The listing builds one solid part. Answer for the finished solid, in the listing's coordinates (mm). A direction names the side the tool comes from. Round coordinates to 2 decimals unless told otherwise and drop trailing zeros. Order: outer loops, then holes, each group sorted by start corner. A loop starts at its lowest first (then second) coordinate and runs counter-clockwise, first axis right, second up. Notation, with made-up numbers: (4.5, -6) - (58.5, -6) arc R13 ccw to (58.5, -2) - close; hole circle Ø1 at (-27, 4.5). An arc over 180 degrees is marked (long way). Use CSV: the item, a comma, the result in double quotes. Start each with the question number.
Item 1: For faces 4 (the flat face through (67, 43.882, 178)), 5 (the flat face through (76, 38.882, 122)), 6 (the flat face through (75, 46, 184.6)), 7 (the flat face through (74, 41.382, 34)), 8 (the flat face through (74, 39, 50)), determine the directions among +Z, -Z, +X, -X, +Y, -Y from which every point of the face is accessible in a straight line to the end or side of a thin tool.
Item 2: Find section C-C, the plane x = 46. Give the vertices of the cut face in (y, z) (3 decimals).
Item 3: Find section B-B, the plane z = 122. Give the vertices of the cut face in (x, y), plus the area to 3 significant figures.
Item 4: Straight lines are drawn through the part: line 1 along X through (y, z) = (37, 50.5); line 2 along X through (y, z) = (39.5, 135); line 3 along Z through (x, y) = (51, 47.25). For each, find the intervals that lie inside material, in ascending order. Write a range as [from, to].
Item 5: Find section A-A, the plane x = 30. Give the vertices of the cut face in (y, z) (3 decimals).
Item 6: Find section D-D, the plane z = -3.5. Give the vertices of the cut face in (x, y).
Item 7: Flat-ended cylindrical pins translate along their axes: P1, Ø3, axis at x = 84.5, y = 40.5, coming from the +Z side; P2, Ø4, axis at x = 121.5, z = 161.17, coming from the +Y side; P3, Ø3.5, axis at x = 66, z = 177.5, coming from the -Y side; P4, Ø0.8, axis at x = 98, y = 39.5, coming from the -Z side. Find the tip coordinate at first contact, or state that the pin passes through.
Item 8: Determine the mould class of faces 1 (the cylindrical face through (119.861, 46.347, 177.936)), 2 (the flat face through (140, 40, 89)), 3 (the cylindrical face through (81.75, 37.952, 176.275)) for opening direction Z: +Z half, -Z half, draft (parallel to the pull), parting line (faces both ways), or undercut.
```python
from build123d import *

# Parameters (mm, degrees)
BOSS_EXTRUDE1_DEPTH     = 150
CUT_EXTRUDE2_REACH      = 244.83
SKETCH2_W               = 50
SKETCH2_H               = 10
FILLET1_R               = 120
SKETCH4_R               = 2.3
BOSS_EXTRUDE2_DEPTH     = 16
SKETCH7_R               = 2.15
CUT_EXTRUDE4_DEPTH      = 11
SKETCH8_W               = 110
SKETCH8_H               = 25
CUT_EXTRUDE5_DEPTH      = 5
CUT_EXTRUDE6_DEPTH      = 2.5
SKETCH10_3_R            = 1.5
CUT_EXTRUDE7_DEPTH      = 239.011365275
FILLET2_R               = 1
CUT_EXTRUDE8_DEPTH      = 239.011365275
CUT_EXTRUDE8_DEPTH_BACK = 239.011365275
SKETCH11_W              = 10
SKETCH11_H              = 194.6


with BuildPart() as part:
    # Sketch1 → Boss-Extrude1 (new body)
    with BuildSketch(Plane(origin=(0, 0, 0), x_dir=(0, 0, -1), z_dir=(1, 0, 0))):
        Polygon((-174.6, 36.381974353), (-174.6, 43.881974353), (-184.6, 43.881974353), (-184.6, 48.881974353), (-169.6, 48.881974353), (-169.6, 41.381974353), (-5, 41.381974353), (-5, 48.881974353), (10, 48.881974353), (10, 43.881974353), (0, 43.881974353), (0, 36.381974353), align=None)
    extrude(amount=BOSS_EXTRUDE1_DEPTH)

    # Sketch2 → Cut-Extrude2 (cut, up to next)
    with BuildSketch(Plane(origin=(0, 0, 0), x_dir=(1, 0, 0), z_dir=(0, 1, 0)), mode=Mode.PRIVATE) as cut_extrude2_sk1:
        with Locations((25, 5)):
            Rectangle(SKETCH2_W, SKETCH2_H)
    cut_extrude2_tool1 = extrude(cut_extrude2_sk1.sketch, amount=CUT_EXTRUDE2_REACH, mode=Mode.PRIVATE) & part.part
    # Sketch2 → Cut-Extrude2 (cut, up to next)
    with BuildSketch(Plane(origin=(0, 0, 0), x_dir=(1, 0, 0), z_dir=(0, 1, 0)), mode=Mode.PRIVATE) as cut_extrude2_sk2:
        with Locations((125, 5)):
            Rectangle(SKETCH2_W, SKETCH2_H)
    cut_extrude2_tool2 = extrude(cut_extrude2_sk2.sketch, amount=CUT_EXTRUDE2_REACH, mode=Mode.PRIVATE) & part.part
    # Sketch2 → Cut-Extrude2 (cut, up to next)
    with BuildSketch(Plane(origin=(0, 0, 0), x_dir=(1, 0, 0), z_dir=(0, 1, 0)), mode=Mode.PRIVATE) as cut_extrude2_sk3:
        with Locations((25, -179.6)):
            Rectangle(SKETCH2_W, SKETCH2_H)
    cut_extrude2_tool3 = extrude(cut_extrude2_sk3.sketch, amount=CUT_EXTRUDE2_REACH, mode=Mode.PRIVATE) & part.part
    # Sketch2 → Cut-Extrude2 (cut, up to next)
    with BuildSketch(Plane(origin=(0, 0, 0), x_dir=(1, 0, 0), z_dir=(0, 1, 0)), mode=Mode.PRIVATE) as cut_extrude2_sk4:
        with Locations((125, -179.6)):
            Rectangle(SKETCH2_W, SKETCH2_H)
    cut_extrude2_tool4 = extrude(cut_extrude2_sk4.sketch, amount=CUT_EXTRUDE2_REACH, mode=Mode.PRIVATE) & part.part
    add(cut_extrude2_tool1.solids().sort_by_distance((25, 0, -5))[0], mode=Mode.SUBTRACT)
    add(cut_extrude2_tool2.solids().sort_by_distance((125, 0, -5))[0], mode=Mode.SUBTRACT)
    add(cut_extrude2_tool3.solids().sort_by_distance((25, 0, 179.6))[0], mode=Mode.SUBTRACT)
    add(cut_extrude2_tool4.solids().sort_by_distance((125, 0, 179.6))[0], mode=Mode.SUBTRACT)

    # Fillet1
    # the kernel refuses this fillet: 120 mm, written as the material it adds along each edge
    with BuildSketch(Plane(origin=(50, 43.881974353, 174.6), x_dir=(-1, 0, 0), z_dir=(0, 1, 0)), Plane(origin=(100, 43.881974353, 0), x_dir=(1, 0, 0), z_dir=(0, 1, 0))) as fillet1_piece_1:
        with BuildLine():
            CenterArc((47.958315233, 120), FILLET1_R, 246.443535691, 23.556464309)
            Line((0, 10), (0, 0))
            Line((0, 0), (47.958315233, 0))
        make_face()
    extrude(amount=5)
    with BuildSketch(Plane(origin=(100, 43.881974353, 174.6), x_dir=(1, 0, 0), z_dir=(0, 1, 0)), Plane(origin=(50, 43.881974353, 0), x_dir=(-1, 0, 0), z_dir=(0, 1, 0))) as fillet1_piece_2:
        with BuildLine():
            CenterArc((47.958315233, -120), FILLET1_R, 90, 23.556464309)
            Line((0, -10), (0, 0))
            Line((0, 0), (47.958315233, 0))
        make_face()
    extrude(amount=5)

    # Sketch4 → Boss-Extrude2 (add)
    with BuildSketch(Plane(origin=(0, 48.881974353, 0), x_dir=(1, 0, 0), z_dir=(0, 1, 0))):
        with Locations(Location((66.85, -178.1, 0), (0, 0, 270))):
            Circle(SKETCH4_R)
        with Locations(Location((83.15, -178.1, 0), (0, 0, 270))):
            Circle(SKETCH4_R)
        with Locations(Location((83.15, 3.5, 0), (0, 0, 270))):
            Circle(SKETCH4_R)
        with Locations(Location((66.85, 3.5, 0), (0, 0, 270))):
            Circle(SKETCH4_R)
    extrude(amount=-BOSS_EXTRUDE2_DEPTH)

    # Sketch7 → Cut-Extrude4 (cut)
    with BuildSketch(Plane.XZ.offset(-32.881974353)):
        with Locations(Location((66.85, 178.1, 0), (0, 0, 270))):
            Circle(SKETCH7_R)
        with Locations(Location((83.15, 178.1, 0), (0, 0, 270))):
            Circle(SKETCH7_R)
        with Locations(Location((66.85, -3.5, 0), (0, 0, 270))):
            Circle(SKETCH7_R)
        with Locations(Location((83.15, -3.5, 0), (0, 0, 270))):
            Circle(SKETCH7_R)
    extrude(amount=-CUT_EXTRUDE4_DEPTH, mode=Mode.SUBTRACT)

    # Sketch8 → Cut-Extrude5 (cut)
    with BuildSketch(Plane(origin=(0, 41.381974353, 0), x_dir=(1, 0, 0), z_dir=(0, 1, 0))):
        with Locations((75, -62.5)):
            Rectangle(SKETCH8_W, SKETCH8_H)
    extrude(amount=-CUT_EXTRUDE5_DEPTH, mode=Mode.SUBTRACT)

    # Sketch10 → Cut-Extrude6 (cut)
    with BuildSketch(Plane(origin=(0, 41.381974353, 0), x_dir=(1, 0, 0), z_dir=(0, 1, 0))):
        Polygon((25, -78.925), (126, -78.925), (126, -165.67443804), (24, -165.67443804), (24, -78.925), align=None)
    extrude(amount=-CUT_EXTRUDE6_DEPTH, mode=Mode.SUBTRACT)

    # Sketch10<3> → Cut-Extrude7 (cut, through all)
    with BuildSketch(Plane(origin=(0, 41.381974353, 0), x_dir=(1, 0, 0), z_dir=(0, 1, 0))):
        with Locations(Location((33.5, -93.425, 0), (0, 0, 270))):
            Circle(SKETCH10_3_R)
        with Locations(Location((121.5, -93.425, 0), (0, 0, 270))):
            Circle(SKETCH10_3_R)
        with Locations(Location((121.5, -161.17443804, 0), (0, 0, 270))):
            Circle(SKETCH10_3_R)
        with Locations(Location((33.5, -161.17443804, 0), (0, 0, 270))):
            Circle(SKETCH10_3_R)
    extrude(amount=-CUT_EXTRUDE7_DEPTH, mode=Mode.SUBTRACT)

    # Fillet2
    fillet2_edges = [part.edges().sort_by_distance(p)[0] for p in [
        (66.85, 43.881974353, 175.8),
        (83.15, 43.881974353, 175.8),
        (83.15, 43.881974353, -5.8),
        (66.85, 43.881974353, -5.8),
    ]]
    fillet(fillet2_edges, radius=FILLET2_R)

    # Sketch11 → Cut-Extrude8 (cut, two sides: drawn at the far end of the back side and taken through both)
    with BuildSketch(Plane(origin=(0, 41.381974353, 0), x_dir=(1, 0, 0), z_dir=(0, 1, 0)).offset(-CUT_EXTRUDE8_DEPTH_BACK)):
        with Locations((5, -87.3)):
            Rectangle(SKETCH11_W, SKETCH11_H)
        with Locations((145, -87.3)):
            Rectangle(SKETCH11_W, SKETCH11_H)
    extrude(amount=CUT_EXTRUDE8_DEPTH + CUT_EXTRUDE8_DEPTH_BACK, mode=Mode.SUBTRACT)


solid = part.part
```
Worked out:
1,face 4,"-Y"
1,face 5,"+Y"
1,face 6,"+Z, +X, -X, +Y, -Y"
1,face 7,"+X, -X, +Y"
1,face 8,"+Y, -Y"
2,outline,"(36.382, 0) - (43.882, 0) - (43.882, -8.341) - (48.882, -8.341) - (48.882, 5) - (41.382, 5) - (41.382, 50) - (36.382, 50) - close; (36.382, 75) - (41.382, 75) - (41.382, 78.925) - (38.882, 78.925) - (38.882, 165.674) - (41.382, 165.674) - (41.382, 169.6) - (48.882, 169.6) - (48.882, 182.941) - (43.882, 182.941) - (43.882, 174.6) - (36.382, 174.6) - close"
3,outline,"(10, 36.38) - (140, 36.38) - (140, 41.38) - (126, 41.38) - (126, 38.88) - (24, 38.88) - (24, 41.38) - (10, 41.38) - close"
3,area,"395 mm²"
4,line 1,"x = [10, 20], [130, 140]"
4,line 2,"x = [10, 24], [126, 140]"
4,line 3,"z = [-10, 5], [169.6, 184.6]"
5,outline,"(36.382, 0) - (43.882, 0) - (43.882, -3.302) - (48.882, -3.302) - (48.882, 5) - (41.382, 5) - (41.382, 50) - (36.382, 50) - close; (36.382, 75) - (41.382, 75) - (41.382, 78.925) - (38.882, 78.925) - (38.882, 165.674) - (41.382, 165.674) - (41.382, 169.6) - (48.882, 169.6) - (48.882, 177.902) - (43.882, 177.902) - (43.882, 174.6) - (36.382, 174.6) - close"
6,outline,"(30.81, 43.88) - (63.55, 43.88) arc R1 cw to (64.55, 42.88) - (64.55, 32.88) - (64.7, 32.88) - (64.7, 43.88) - (69, 43.88) - (69, 32.88) - (69.15, 32.88) - (69.15, 42.88) arc R1 cw to (70.15, 43.88) - (79.85, 43.88) arc R1 cw to (80.85, 42.88) - (80.85, 32.88) - (81, 32.88) - (81, 43.88) - (85.3, 43.88) - (85.3, 32.88) - (85.45, 32.88) - (85.45, 42.88) arc R1 cw to (86.45, 43.88) - (119.19, 43.88) - (119.19, 48.88) - (30.81, 48.88) - close"
7,P1,"stops at z = 180.4"
7,P2,"stops at y = 38.88"
7,P3,"stops at y = 32.88"
7,P4,"stops at z = 0"
8,face 1,"+Z half"
8,face 2,"draft"
8,face 3,"undercut"
